Drawing for the job (mm, zero at the part's lowest x, y, z). A direction names the side the tool comes from. Coordinates: 2 decimals unless noted, no trailing zeros. Write each loop counter-clockwise with the first axis right and the second up, starting at its lowest first coordinate (ties: lowest second). Pieces come first, ordered by that corner, then holes. Notation, with made-up numbers: (70.25, 53.5) -> (74.25, 53.5) arc R34 cw to (74.25, 84.5) -> close; hole circle Ø2 at (57.25, -1). An arc over 180 degrees is marked (long way). Answer as CSV lines item,"result". Start each with the question number.
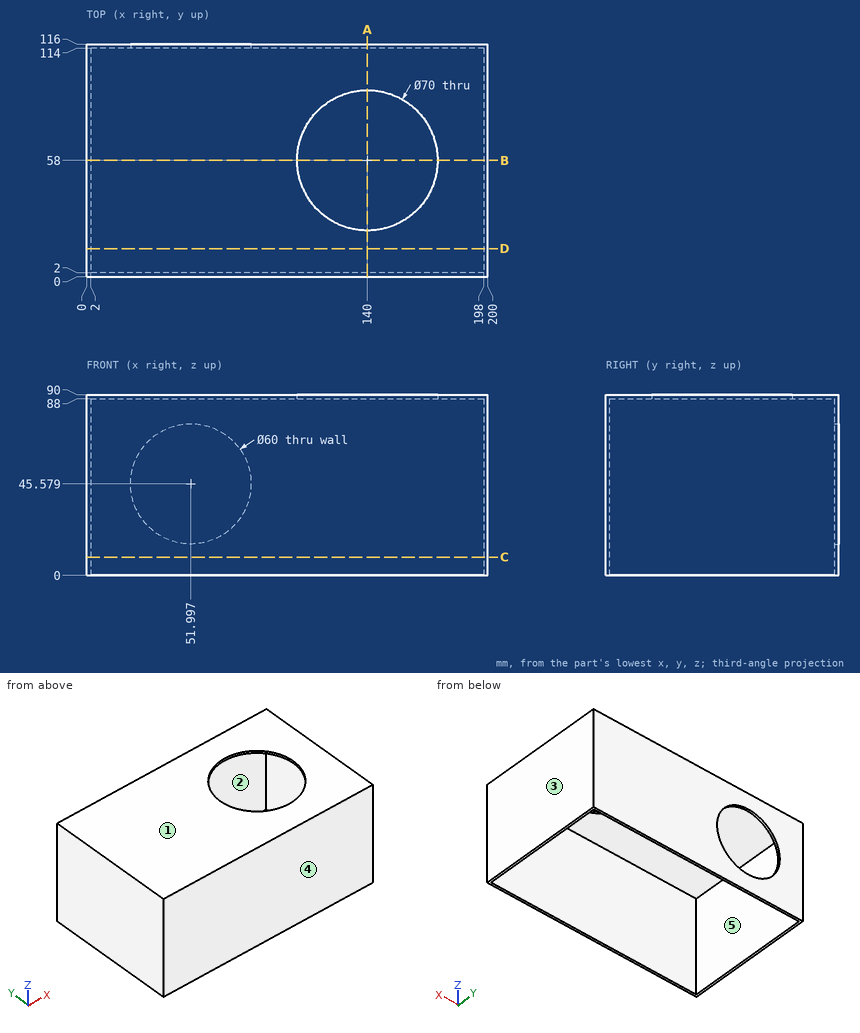
1. Wall check: line 1 (X direction, y = 83, z = 59); line 2 (Y direction, x = 151.5, z = 73); line 3 (Z direction, x = 55.5, y = 25). Give the ranges that are in metal, low to high.
2. Cut at B-B (y = 58). Give the cut face in (x, z), then the cut area to 3 significant figures.
3. Cut at C-C (z = 9). Give the cut face in (x, y).
4. Mould opens along X. For the marked faces 1, 2 and 3 say: pulls with the +X half, pulls with the -X half, needs draft (parallel to the pull), parting line crosses it, or undercut.
5. Cut at A-A (x = 140). Give the cut face in (y, z).
6. Cut at D-D (y = 14). Give the cut face in (x, z).
7. Tool access for the marked faces 4 and 5: list every direction of +Z, -Z, +X, -X, +Y, -Y with a clear straight run to the whole face (end or side of a thin tool).
Geometry check:
1,line 1,"0 to 2, 198 to 200"
1,line 2,"0 to 2, 114 to 116"
1,line 3,"88 to 90"
2,outline,"(0, 0) -> (2, 0) -> (2, 88) -> (105, 88) -> (105, 90) -> (0, 90) -> close; (175, 88) -> (198, 88) -> (198, 0) -> (200, 0) -> (200, 90) -> (175, 90) -> close"
2,area,"612 mm²"
3,outline,"(0, 0) -> (200, 0) -> (200, 116) -> (0, 116) -> close; hole (2, 2) -> (198, 2) -> (198, 114) -> (2, 114) -> close"
4,face 1,"needs draft"
4,face 2,"undercut"
4,face 3,"pulls with the +X half"
5,outline,"(0, 0) -> (2, 0) -> (2, 88) -> (23, 88) -> (23, 90) -> (0, 90) -> close; (93, 88) -> (114, 88) -> (114, 0) -> (116, 0) -> (116, 90) -> (93, 90) -> close"
6,outline,"(0, 0) -> (2, 0) -> (2, 88) -> (198, 88) -> (198, 0) -> (200, 0) -> (200, 90) -> (0, 90) -> close"
7,face 4,"+Z, -Z, +X, -X, -Y"
7,face 5,"-Z"
